Check sheet for the drawn part. Datum: minimum x, y, z corner. Units: mm. A direction names the side the tool comes from. Coordinates: 2 decimals unless noted, no trailing zeros. Write each loop counter-clockwise with the first axis right and the second up, starting at its lowest first coordinate (ties: lowest second). Pieces come first, ordered by that corner, then holes. Notation, with made-up numbers: M 1,87.5 L 35,87.5 A20 ccw 35,117.5 Z; hole C 45.5,81.25 d10. An arc over 180 degrees is marked long. Answer in a Markdown table with one row per item.
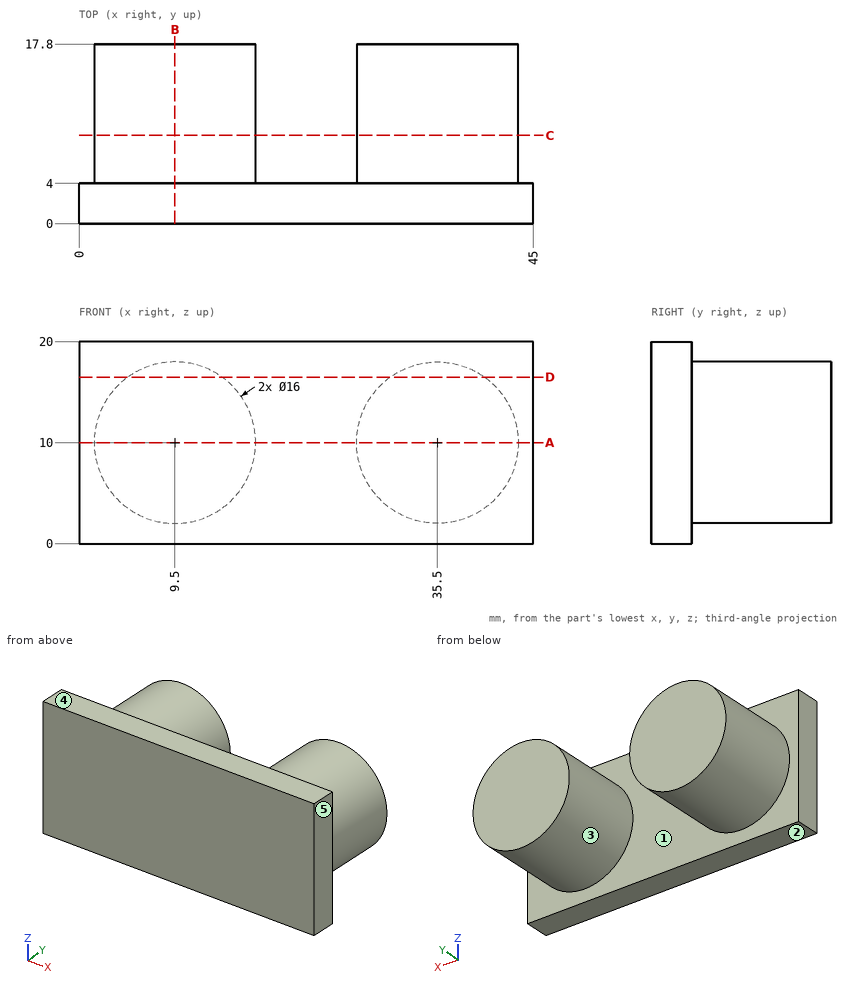
1) Sectioned sample at B-B (x = 9.5). Record the cut outline in (y, z).
Response values:
| item | result |
|---|---|
| outline | M 0,0 L 4,0 L 4,2 L 17.8,2 L 17.8,18 L 4,18 L 4,20 L 0,20 Z |
2) Sectioned sample at C-C (y = 8.75). Record the cut outline in (x, z).
Response values:
| item | result |
|---|---|
| outline | C 9.5,10 d16; C 35.5,10 d16 |
3) Sectioned sample at A-A (z = 10). Record the cut outline in (x, y), then the cut area to 3 significant figures.
Response values:
| item | result |
|---|---|
| outline | M 0,0 L 45,0 L 45,4 L 43.5,4 L 43.5,17.8 L 27.5,17.8 L 27.5,4 L 17.5,4 L 17.5,17.8 L 1.5,17.8 L 1.5,4 L 0,4 Z |
| area | 622 mm² |
4) Depth check by flat-ended pin: pin 1 (1.5 mm diameter, centred on x = 30, y = 3.5, fed in from -Z); pin 2 (1.5 mm diameter, centred on x = 14, y = 7.5, fed in from +Z); pin 3 (4 mm diameter, centred on x = 11, y = 13, fed in from -Z); pin 4 (1.5 mm diameter, centred on x = 6.5, y = 6, fed in from +Z). Enter the tip coordinate at first touch or a pass-through.
Response values:
| item | result |
|---|---|
| pin 1 | stops at z = 0 |
| pin 2 | stops at z = 17.07 |
| pin 3 | stops at z = 2 |
| pin 4 | stops at z = 17.68 |
5) Release check for a two-part mould opening along X. For the marked faces 3, 4 and 5 record: +X half, -X half, draft (parallel to the pull), parting line (faces both ways), or undercut.
Response values:
| item | result |
|---|---|
| face 3 | undercut |
| face 4 | draft |
| face 5 | +X half |
6) Tool access check on the marked faces 1 and 2. Record the directions out of +Z, -Z, +X, -X, +Y, -Y that give a thin tool (end or side, any length) a straight path to the whole face; none if there is none.
Response values:
| item | result |
|---|---|
| face 1 | +Y |
| face 2 | -Z, +X, -X, +Y, -Y |
7) Thickness scan on L1, parallel to Y at x = 30.5, z = 17; L2, parallel to X at y = 11.75, z = 7; L3, parallel to X at y = 8.5, z = 6. Record the ranges inside material, lowest first. Write a range as [from, to].
Response values:
| item | result |
|---|---|
| L1 | y = [0, 4] |
| L2 | x = [2.08, 16.92], [28.08, 42.92] |
| L3 | x = [2.57, 16.43], [28.57, 42.43] |
8) Sectioned sample at D-D (z = 16.5). Record the cut outline in (x, y).
Response values:
| item | result |
|---|---|
| outline | M 0,0 L 45,0 L 45,4 L 40.16,4 L 40.16,17.8 L 30.84,17.8 L 30.84,4 L 14.16,4 L 14.16,17.8 L 4.84,17.8 L 4.84,4 L 0,4 Z |
